```python
from build123d import *

# Parameters (mm, degrees)
FILLET_1_R          = 0.2
CUT_EXTRUDE_1_DEPTH = 1.5
SKETCH_3_R          = 1.5
EXTRUDE_1_DEPTH     = 8
CHAMFER_1_SIZE      = 0.5


with BuildPart() as part:
    # 草图1 → 旋转1 (revolve)
    with BuildSketch(Plane.XY):
        with BuildLine():
            Line((0, 0), (0, 2))
            Line((0, 2), (1.3, 2))
            ThreePointArc((1.3, 2), (2.370691821, 1.250626571), (2.75, 0))
            Line((2.75, 0), (0, 0))
        make_face()
    revolve(axis=Axis((0, 0, 0), (0, 1, 0)))

    # 圆角1
    fillet_1_edges = [part.edges().sort_by_distance(p)[0] for p in [
        (-2.75, 0, 0),
    ]]
    fillet(fillet_1_edges, radius=FILLET_1_R)

    # 草图2 → 切除-拉伸1 (cut)
    with BuildSketch(Plane(origin=(0, 2, 0), x_dir=(1, 0, 0), z_dir=(0, 1, 0))):
        Polygon((1.327905619, 0), (0.66395281, 1.15), (-0.66395281, 1.15), (-1.327905619, 0), (-0.66395281, -1.15), (0.66395281, -1.15), align=None)
    extrude(amount=-CUT_EXTRUDE_1_DEPTH, mode=Mode.SUBTRACT)

    # 草图3 → 凸台-拉伸1 (add)
    with BuildSketch(Plane.XZ):
        Circle(SKETCH_3_R)
    extrude(amount=EXTRUDE_1_DEPTH)

    # 倒角1
    chamfer_1_edges = [part.edges().sort_by_distance(p)[0] for p in [
        (-1.5, -8, 0),
    ]]
    chamfer(chamfer_1_edges, length=CHAMFER_1_SIZE)


solid = part.part
```
CAD build for the part. Positions are in the model's coordinates, mm. A direction names the side the tool comes from. Coordinates: 2 decimals unless noted, no trailing zeros. Order: outer loops, then holes, each group sorted by start corner. A loop starts at its lowest first (then second) coordinate and runs counter-clockwise, first axis right, second up.
(1) Saw through at A-A, the plane y = -5. Write the cut outline in (x, z), and give its area (3 significant figures).
Solution:
outline: circle Ø3 at (0, 0)
area: 7.07 mm2
(2) Which spindle directions (+Z, -Z, +X, -X, +Y, -Y) get a long thin tool onto all of the face, cutting with end or side? Do faces 1 (the face through (0, -8, 0)), 2 (the face through (1, 1.26, -0.57)). Say none if no direction does.
Solution:
face 1: +Z, -Z, +X, -X, -Y
face 2: +Y
(3) Pin check, flat tips, straight feed: pin 1 Ø3 at (x, y) = (-0.5, -3.5) entering from -Z; pin 2 Ø3 at (x, y) = (-2, -2.5) entering from +Z; pin 3 Ø0.7 at (x, y) = (-0.5, 1.5) entering from -Z. Stop position of each tip, or through.
Solution:
pin 1: stops at z = -1.5
pin 2: stops at z = 1.41
pin 3: stops at z = -2.4
(4) Mould opens along X. For faces 3 (the face through (-1.5, -3.7, 0.07)), 4 (the face through (0, 0, 2)), 5 (the face through (0, 0.5, 0)) say: released by +X, released by -X, zero draft, split by the parting line, or undercut.
Solution:
face 3: split by the parting line
face 4: zero draft
face 5: undercut
(5) Drill centre lines: L1, parallel to Y at x = 0.05, z = -0.6; L2, parallel to Z at x = 0.6, y = 1.25; L3, parallel to Z at x = 0.1, y = -4. Where is each one in solid material? Low to high.
Solution:
L1: y = -8 to 0.5
L2: z = -2.29 to -1.15, 1.15 to 2.29
L3: z = -1.5 to 1.5
